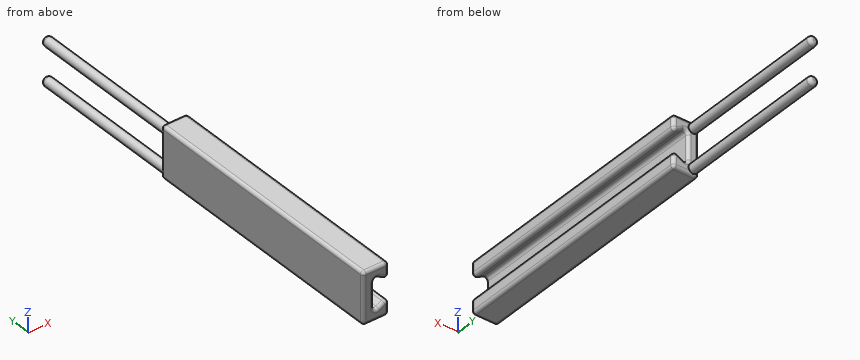
```python
from build123d import *
from OCP.BRepFilletAPI import BRepFilletAPI_MakeFillet

# Parameters (mm, degrees)
BOSS_EXTRUDE2_DEPTH      = 127
FILLET1_R1               = 1.5875
FILLET1_R2               = 1.4732
BOSS_EXTRUDE3_DEPTH      = 76.2
BOSS_EXTRUDE3_DEPTH_BACK = 2.54
SKETCH2_R                = 2.286
FILLET2_R                = 1.778


with BuildPart() as part:
    # Sketch1 → Boss-Extrude2 (new body)
    with BuildSketch(Plane(origin=(0, 0, 0), x_dir=(1, 0, 0), z_dir=(0, 1, 0))):
        Polygon((-28.067579909, 0), (-28.067579909, -25.4), (-15.367579909, -25.4), (-15.367579909, -16.933333333), (-22.699928279, -21.166666582), (-22.699928279, -4.233333249), (-15.367579909, -8.466666667), (-15.367579909, 0), align=None)
    extrude(amount=BOSS_EXTRUDE2_DEPTH)

    # Fillet1: one fillet with a radius per group of edges: ONE call of the kernel's fillet builder (fillet() takes one radius for all edges)
    fillet1_edges_1 = [part.edges().sort_by_distance(p)[0] for p in [
        (-19.033754094, 127, 6.349999958),
        (-22.699928279, 127, 12.699999915),
        (-19.033754094, 127, 19.049999958),
        (-15.367579909, 127, 21.166666667),
        (-15.367579909, 127, 4.233333333),
        (-21.717579909, 127, 0),
        (-28.067579909, 63.5, 0),
        (-15.367579909, 63.5, 0),
        (-21.717579909, 0, 0),
        (-15.367579909, 0, 4.233333333),
        (-15.367579909, 63.5, 8.466666667),
        (-15.367579909, 63.5, 16.933333333),
        (-15.367579909, 0, 21.166666667),
        (-15.367579909, 63.5, 25.4),
        (-22.699928279, 0, 12.699999915),
        (-28.067579909, 127, 12.7),
        (-21.717579909, 127, 25.4),
        (-28.067579909, 63.5, 25.4),
        (-28.067579909, 0, 12.7),
        (-21.717579909, 0, 25.4),
        (-19.033754094, 0, 6.349999958),
        (-19.033754094, 0, 19.049999958),
    ]]
    fillet1_edges_2 = [part.edges().sort_by_distance(p)[0] for p in [
        (-22.699928279, 63.5, 4.233333249),
        (-22.699928279, 63.5, 21.166666582),
    ]]
    fillet1 = BRepFilletAPI_MakeFillet(part.part.solid().wrapped)
    for e in fillet1_edges_1:
        fillet1.Add(FILLET1_R1, e.wrapped)
    for e in fillet1_edges_2:
        fillet1.Add(FILLET1_R2, e.wrapped)
    add(Compound.cast(fillet1.Shape()), mode=Mode.REPLACE)

    # Sketch2 → Boss-Extrude3 (add, two sides: drawn at the far end of the back side and taken through both)
    with BuildSketch(Plane(origin=(0, 127, 0), x_dir=(1, 0, 0), z_dir=(0, 1, 0)).offset(-BOSS_EXTRUDE3_DEPTH_BACK)):
        with Locations(Location((-25.235504788, -3.154170131, 0), (0, 0, 270))):
            Circle(SKETCH2_R)
        with Locations(Location((-25.235504788, -22.245829751, 0), (0, 0, 237.01403639))):
            Circle(SKETCH2_R)
    extrude(amount=BOSS_EXTRUDE3_DEPTH + BOSS_EXTRUDE3_DEPTH_BACK)

    # Fillet2
    fillet2_edges = [part.edges().sort_by_distance(p)[0] for p in [
        (-23.99092967, 203.2, 20.328323877),
        (-25.235504788, 203.2, 0.868170131),
    ]]
    fillet(fillet2_edges, radius=FILLET2_R)


solid = part.part
```
Check sheet for the modelled part. Datum: model origin and axes. Units: mm. Round coordinates to 2 decimals unless told otherwise and drop trailing zeros. Loops run counter-clockwise (first coordinate to the right, second up) from the corner with the lowest first, then second, coordinate; pieces in that order, holes last. Notation, with made-up numbers: (-33, 41.5) - (2, 41.5) arc R20 ccw to (2, 57.5) - close; hole circle Ø1 at (87.5, -29.5). An arc over 180 degrees is marked (long way). Write item = value, one per line. Start each with the question number.
Q1. Section check B-B (y = 16). Record the boundary of the cut face in (x, z) (1 decimal), plus the area to 3 significant figures.
Q2. Section check A-A (z = 14.5). Record the boundary of the cut face in (x, y) (1 decimal), plus the area to 3 significant figures.
Q3. Thickness scan on L1, parallel to Z at x = -22, y = 117.5; L2, parallel to Z at x = -22.25, y = 96; L3, parallel to X at y = 119, z = 10.75. Record the ranges inside material, lowest first.
Q4. Section check C-C (y = 154.5). Record the boundary of the cut face in (x, z).
Q5. Depth check by flat-ended pin: P1, Ø7.5, axis at x = -22, z = 11, coming from the +Y side; P2, Ø3, axis at y = 88, z = 10, coming from the +X side. Enter the tip coordinate at first touch or a pass-through.
Derived:
q1.outline = (-28.1, 1.6) arc R1.6 ccw to (-26.5, 0) - (-17, 0) arc R1.6 ccw to (-15.4, 1.6) - (-15.4, 5.7) arc R1.6 ccw to (-17.7, 7.1) - (-20.5, 5.5) arc R1.5 cw to (-22.7, 6.8) - (-22.7, 18.6) arc R1.5 cw to (-20.5, 19.9) - (-17.7, 18.3) arc R1.6 ccw to (-15.4, 19.7) - (-15.4, 23.8) arc R1.6 ccw to (-17, 25.4) - (-26.5, 25.4) arc R1.6 ccw to (-28.1, 23.8) - close
q1.area = 227 mm^2
q2.outline = (-28.1, 1.6) arc R1.6 ccw to (-26.5, 0) - (-24.3, 0) arc R1.6 ccw to (-22.7, 1.6) - (-22.7, 125.4) arc R1.6 ccw to (-24.3, 127) - (-26.5, 127) arc R1.6 ccw to (-28.1, 125.4) - close
q2.area = 680 mm^2
q3.L1 = 0 to 5.53, 19.87 to 25.4
q3.L2 = 0 to 5.73, 19.67 to 25.4
q3.L3 = -28.07 to -22.7
q4.outline = circle Ø4.57 at (-25.24, 3.15); circle Ø4.57 at (-25.24, 22.25)
q5.P1 = 127
q5.P2 = -22.7
